```python
from build123d import *

# Parameters (mm, degrees)
SKETCH_1_R               = 45
SKETCH_1_R_2             = 1
SKETCH_1_R_3             = 35
EXTRUDE_2_DEPTH          = 14.9
EXTRUDE_START            = -4
SKETCH_3_R               = 47.8
SKETCH_3_R_2             = 45
EXTRUDE_3_DEPTH          = 4
PATTERN_CIRCULAR_1_COUNT = 8
CUT_EXTRUDE_2_DEPTH      = 12
SKETCH_14_R              = 47.8
SKETCH_14_R_2            = 45
CUT_EXTRUDE_3_DEPTH      = 10
SKETCH_15_R              = 47.8
SKETCH_15_R_2            = 45
EXTRUDE_4_DEPTH          = 7
CUT_EXTRUDE_4_DEPTH      = 10


with BuildPart() as part:
    # Sketch 1 → Extrude 2 (new body)
    with BuildSketch(Plane.XY):
        Circle(SKETCH_1_R)
        with Locations((0, 40)):
            Circle(SKETCH_1_R_2, mode=Mode.SUBTRACT)
        with Locations((28.284271247, 28.284271247)):
            Circle(SKETCH_1_R_2, mode=Mode.SUBTRACT)
        with Locations((40, 0)):
            Circle(SKETCH_1_R_2, mode=Mode.SUBTRACT)
        with Locations((28.284271247, -28.284271247)):
            Circle(SKETCH_1_R_2, mode=Mode.SUBTRACT)
        with Locations((0, -40)):
            Circle(SKETCH_1_R_2, mode=Mode.SUBTRACT)
        with Locations((-28.284271247, -28.284271247)):
            Circle(SKETCH_1_R_2, mode=Mode.SUBTRACT)
        Circle(SKETCH_1_R_3, mode=Mode.SUBTRACT)
        with Locations((-40, 0)):
            Circle(SKETCH_1_R_2, mode=Mode.SUBTRACT)
        with Locations((-28.284271247, 28.284271247)):
            Circle(SKETCH_1_R_2, mode=Mode.SUBTRACT)
    extrude(amount=EXTRUDE_2_DEPTH)

    # Sketch 3 → Extrude 3 (add)
    with BuildSketch(Plane.XY.offset(14.9).offset(EXTRUDE_START)):
        Circle(SKETCH_3_R)
        Circle(SKETCH_3_R_2, mode=Mode.SUBTRACT)
    extrude(amount=EXTRUDE_3_DEPTH)

    # Sketch 12 → Hole Wizard M5 _1 (revolve, cut)
    with BuildSketch(Plane(origin=(0, 40, 0), x_dir=(0, 1, 0), z_dir=(1, 0, 0))):
        Polygon((0, 0), (0, 23.6618073), (2.1, 22.4), (2.1, 0), align=None)
    hole_wizard_m5_1 = revolve(axis=Axis((0, 40, -6.35), (0, 0, 1)), mode=Mode.SUBTRACT)

    # Pattern Circular 1: Hole Wizard M5 _1 ×8 about axis
    pattern_circular_1_axis = Axis((0, 0, 0), (0, 0, 1))
    for i in range(1, PATTERN_CIRCULAR_1_COUNT):
        add(hole_wizard_m5_1.rotate(pattern_circular_1_axis, i * 360 / PATTERN_CIRCULAR_1_COUNT), mode=Mode.SUBTRACT)

    # Sketch 13 → Cut-Extrude 2 (cut)
    with BuildSketch(Plane(origin=(0, 0, 0), x_dir=(-1, 0, 0), z_dir=(0, 0, -1))):
        with BuildLine():
            ThreePointArc((-8.473137213, 41.646799946), (-16.264045876, 39.264880132), (-23.457321876, 35.440147438))
            ThreePointArc((-23.457321876, 35.440147438), (-24.162193968, 31.975590419), (-20.697636949, 31.270718328))
            ThreePointArc((-20.697636949, 31.270718328), (-14.350628714, 34.645482469), (-7.476297541, 36.747176423))
            ThreePointArc((-7.476297541, 36.747176423), (-5.524905615, 39.695408021), (-8.473137213, 41.646799946))
        make_face()
        with BuildLine():
            ThreePointArc((23.457321876, 35.440147438), (16.264045876, 39.264880132), (8.473137213, 41.646799946))
            ThreePointArc((8.473137213, 41.646799946), (5.524905615, 39.695408021), (7.476297541, 36.747176423))
            ThreePointArc((7.476297541, 36.747176423), (14.350628714, 34.645482469), (20.697636949, 31.270718328))
            ThreePointArc((20.697636949, 31.270718328), (24.162193968, 31.975590419), (23.457321876, 35.440147438))
        make_face()
        with BuildLine():
            ThreePointArc((41.646799946, 8.473137213), (39.264880132, 16.264045876), (35.440147438, 23.457321876))
            ThreePointArc((35.440147438, 23.457321876), (31.975590419, 24.162193968), (31.270718328, 20.697636949))
            ThreePointArc((31.270718328, 20.697636949), (34.645482469, 14.350628714), (36.747176423, 7.476297541))
            ThreePointArc((36.747176423, 7.476297541), (39.695408021, 5.524905615), (41.646799946, 8.473137213))
        make_face()
        with BuildLine():
            ThreePointArc((35.440147438, -23.457321876), (39.264880132, -16.264045876), (41.646799946, -8.473137213))
            ThreePointArc((41.646799946, -8.473137213), (39.695408021, -5.524905615), (36.747176423, -7.476297541))
            ThreePointArc((36.747176423, -7.476297541), (34.645482469, -14.350628714), (31.270718328, -20.697636949))
            ThreePointArc((31.270718328, -20.697636949), (31.975590419, -24.162193968), (35.440147438, -23.457321876))
        make_face()
        with BuildLine():
            ThreePointArc((8.473137213, -41.646799946), (16.264045876, -39.264880132), (23.457321876, -35.440147438))
            ThreePointArc((23.457321876, -35.440147438), (24.162193968, -31.975590419), (20.697636949, -31.270718328))
            ThreePointArc((20.697636949, -31.270718328), (14.350628714, -34.645482469), (7.476297541, -36.747176423))
            ThreePointArc((7.476297541, -36.747176423), (5.524905615, -39.695408021), (8.473137213, -41.646799946))
        make_face()
        with BuildLine():
            ThreePointArc((-23.457321876, -35.440147438), (-16.264045876, -39.264880132), (-8.473137213, -41.646799946))
            ThreePointArc((-8.473137213, -41.646799946), (-5.524905615, -39.695408021), (-7.476297541, -36.747176423))
            ThreePointArc((-7.476297541, -36.747176423), (-14.350628714, -34.645482469), (-20.697636949, -31.270718328))
            ThreePointArc((-20.697636949, -31.270718328), (-24.162193968, -31.975590419), (-23.457321876, -35.440147438))
        make_face()
        with BuildLine():
            ThreePointArc((-41.646799946, -8.473137213), (-39.264880132, -16.264045876), (-35.440147438, -23.457321876))
            ThreePointArc((-35.440147438, -23.457321876), (-31.975590419, -24.162193968), (-31.270718328, -20.697636949))
            ThreePointArc((-31.270718328, -20.697636949), (-34.645482469, -14.350628714), (-36.747176423, -7.476297541))
            ThreePointArc((-36.747176423, -7.476297541), (-39.695408021, -5.524905615), (-41.646799946, -8.473137213))
        make_face()
        with BuildLine():
            ThreePointArc((-35.440147438, 23.457321876), (-39.264880132, 16.264045876), (-41.646799946, 8.473137213))
            ThreePointArc((-41.646799946, 8.473137213), (-39.695408021, 5.524905615), (-36.747176423, 7.476297541))
            ThreePointArc((-36.747176423, 7.476297541), (-34.645482469, 14.350628714), (-31.270718328, 20.697636949))
            ThreePointArc((-31.270718328, 20.697636949), (-31.975590419, 24.162193968), (-35.440147438, 23.457321876))
        make_face()
    extrude(amount=-CUT_EXTRUDE_2_DEPTH, mode=Mode.SUBTRACT)

    # Sketch 14 → Cut-Extrude 3 (cut)
    with BuildSketch(Plane(origin=(0, 0, 10.9), x_dir=(-1, 0, 0), z_dir=(0, 0, -1))):
        Circle(SKETCH_14_R)
        with Locations(Location((0, 0, 0), (0, 0, 180))):
            Circle(SKETCH_14_R_2, mode=Mode.SUBTRACT)
    extrude(amount=-CUT_EXTRUDE_3_DEPTH, mode=Mode.SUBTRACT)

    # Sketch 15 → Extrude 4 (add)
    with BuildSketch(Plane(origin=(0, 0, 0), x_dir=(-1, 0, 0), z_dir=(0, 0, -1))):
        Circle(SKETCH_15_R)
        Circle(SKETCH_15_R_2, mode=Mode.SUBTRACT)
    extrude(amount=-EXTRUDE_4_DEPTH)

    # Sketch 16 → Cut-Extrude 4 (cut)
    with BuildSketch(Plane(origin=(0, 0, 12), x_dir=(-1, 0, 0), z_dir=(0, 0, -1))):
        with BuildLine():
            ThreePointArc((-20.697636949, -31.270718328), (-24.162193968, -31.975590419), (-23.457321876, -35.440147438))
            ThreePointArc((-23.457321876, -35.440147438), (-16.264045876, -39.264880132), (-8.473137213, -41.646799946))
            ThreePointArc((-8.473137213, -41.646799946), (-5.524905615, -39.695408021), (-7.476297541, -36.747176423))
            ThreePointArc((-7.476297541, -36.747176423), (-14.350628714, -34.645482469), (-20.697636949, -31.270718328))
        make_face()
        with BuildLine():
            ThreePointArc((7.476297541, -36.747176423), (5.524905615, -39.695408021), (8.473137213, -41.646799946))
            ThreePointArc((8.473137213, -41.646799946), (16.264045876, -39.264880132), (23.457321876, -35.440147438))
            ThreePointArc((23.457321876, -35.440147438), (24.162193968, -31.975590419), (20.697636949, -31.270718328))
            ThreePointArc((20.697636949, -31.270718328), (14.350628714, -34.645482469), (7.476297541, -36.747176423))
        make_face()
        with BuildLine():
            ThreePointArc((31.270718328, -20.697636949), (31.975590419, -24.162193968), (35.440147438, -23.457321876))
            ThreePointArc((35.440147438, -23.457321876), (39.264880132, -16.264045876), (41.646799946, -8.473137213))
            ThreePointArc((41.646799946, -8.473137213), (39.695408021, -5.524905615), (36.747176423, -7.476297541))
            ThreePointArc((36.747176423, -7.476297541), (34.645482469, -14.350628714), (31.270718328, -20.697636949))
        make_face()
        with BuildLine():
            ThreePointArc((36.747176423, 7.476297541), (39.695408021, 5.524905615), (41.646799946, 8.473137213))
            ThreePointArc((41.646799946, 8.473137213), (39.264880132, 16.264045876), (35.440147438, 23.457321876))
            ThreePointArc((35.440147438, 23.457321876), (31.975590419, 24.162193968), (31.270718328, 20.697636949))
            ThreePointArc((31.270718328, 20.697636949), (34.645482469, 14.350628714), (36.747176423, 7.476297541))
        make_face()
        with BuildLine():
            ThreePointArc((20.697636949, 31.270718328), (24.162193968, 31.975590419), (23.457321876, 35.440147438))
            ThreePointArc((23.457321876, 35.440147438), (16.264045876, 39.264880132), (8.473137213, 41.646799946))
            ThreePointArc((8.473137213, 41.646799946), (5.524905615, 39.695408021), (7.476297541, 36.747176423))
            ThreePointArc((7.476297541, 36.747176423), (14.350628714, 34.645482469), (20.697636949, 31.270718328))
        make_face()
        with BuildLine():
            ThreePointArc((-7.476297541, 36.747176423), (-5.524905615, 39.695408021), (-8.473137213, 41.646799946))
            ThreePointArc((-8.473137213, 41.646799946), (-16.264045876, 39.264880132), (-23.457321876, 35.440147438))
            ThreePointArc((-23.457321876, 35.440147438), (-24.162193968, 31.975590419), (-20.697636949, 31.270718328))
            ThreePointArc((-20.697636949, 31.270718328), (-14.350628714, 34.645482469), (-7.476297541, 36.747176423))
        make_face()
        with BuildLine():
            ThreePointArc((-31.270718328, 20.697636949), (-31.975590419, 24.162193968), (-35.440147438, 23.457321876))
            ThreePointArc((-35.440147438, 23.457321876), (-39.264880132, 16.264045876), (-41.646799946, 8.473137213))
            ThreePointArc((-41.646799946, 8.473137213), (-39.695408021, 5.524905615), (-36.747176423, 7.476297541))
            ThreePointArc((-36.747176423, 7.476297541), (-34.645482469, 14.350628714), (-31.270718328, 20.697636949))
        make_face()
        with BuildLine():
            ThreePointArc((-36.747176423, -7.476297541), (-39.695408021, -5.524905615), (-41.646799946, -8.473137213))
            ThreePointArc((-41.646799946, -8.473137213), (-39.264880132, -16.264045876), (-35.440147438, -23.457321876))
            ThreePointArc((-35.440147438, -23.457321876), (-31.975590419, -24.162193968), (-31.270718328, -20.697636949))
            ThreePointArc((-31.270718328, -20.697636949), (-34.645482469, -14.350628714), (-36.747176423, -7.476297541))
        make_face()
    extrude(amount=-CUT_EXTRUDE_4_DEPTH, mode=Mode.SUBTRACT)


solid = part.part
```
For this review, take the finished solid that the model builds, in its own axes (mm). Coordinates: 2 decimals unless noted, no trailing zeros. Order: outer loops, then holes, each group sorted by start corner. A loop starts at its lowest first (then second) coordinate and runs counter-clockwise, first axis right, second up. Notation, with made-up numbers: (12.25, -8) -> (19.25, -8) arc R23 cw to (19.25, 15) -> close; hole circle Ø1 at (21, -31). An arc over 180 degrees is marked (long way). Use CSV: the item, a comma, the result in double quotes. Start each with the question number.
Item 1: Insertion check: pin 1 (4 mm diameter, centred on y = 25.5, z = 13, fed in from -X); pin 2 (3 mm diameter, centred on y = 25.5, z = 13, fed in from +X); pin 3 (4 mm diameter, centred on x = 31, z = 2.5, fed in from -Y). Each pin has a flat end and moves straight along its axis. Give the tip position at first contact, or say it passes through.
Item 2: We need section C-C, the plane z = 10. Give the number of separate pieces and of enclosed holes in the cut face, then the cut area to 3 significant figures.
Item 3: We need section A-A, the plane y = 0. Give the boundary of the cut face in (x, z).
Item 4: Draft analysis for pull direction Y (two halves, no side actions). For faces 1 (the face through (32, -32, 7)), 2 (the face through (24.13, -31.93, 7.35)), 3 (the face through (20.765, -39.923, 10.895)), state which applies: pulls with the +Y half, pulls with the -Y half, needs draft (parallel to the pull), parting line crosses it, or undercut.
Item 5: Wall thickness on probe 1 along Y at (x, z) = (0, 6); probe 2 along Y at (x, z) = (0, 12); probe 3 along X at (y, z) = (-11, 7.25): over which ranges is each line inside the solid? List them lowest first.
Derived:
1,pin 1,"stops at x = -38.38"
1,pin 2,"stops at x = 38.07"
1,pin 3,"stops at y = -38"
2,separate pieces,"1"
2,enclosed holes,"17"
2,area,"1,630 mm^2"
3,outline,"(-47.8, 0) -> (-42.1, 0) -> (-42.1, 14.9) -> (-45, 14.9) -> (-45, 7) -> (-47.8, 7) -> close; (-37.9, 0) -> (-35, 0) -> (-35, 14.9) -> (-37.9, 14.9) -> close; (35, 0) -> (37.9, 0) -> (37.9, 14.9) -> (35, 14.9) -> close; (42.1, 0) -> (47.8, 0) -> (47.8, 7) -> (45, 7) -> (45, 14.9) -> (42.1, 14.9) -> close"
4,face 1,"needs draft"
4,face 2,"undercut"
4,face 3,"parting line crosses it"
5,probe 1,"y = -47.8 to -42.1, -37.9 to -35, 35 to 37.9, 42.1 to 47.8"
5,probe 2,"y = -45 to -42.1, -37.9 to -35, 35 to 37.9, 42.1 to 45"
5,probe 3,"x = -43.63 to -41.05, -35.85 to -33.23, 33.23 to 35.85, 41.05 to 43.63"
